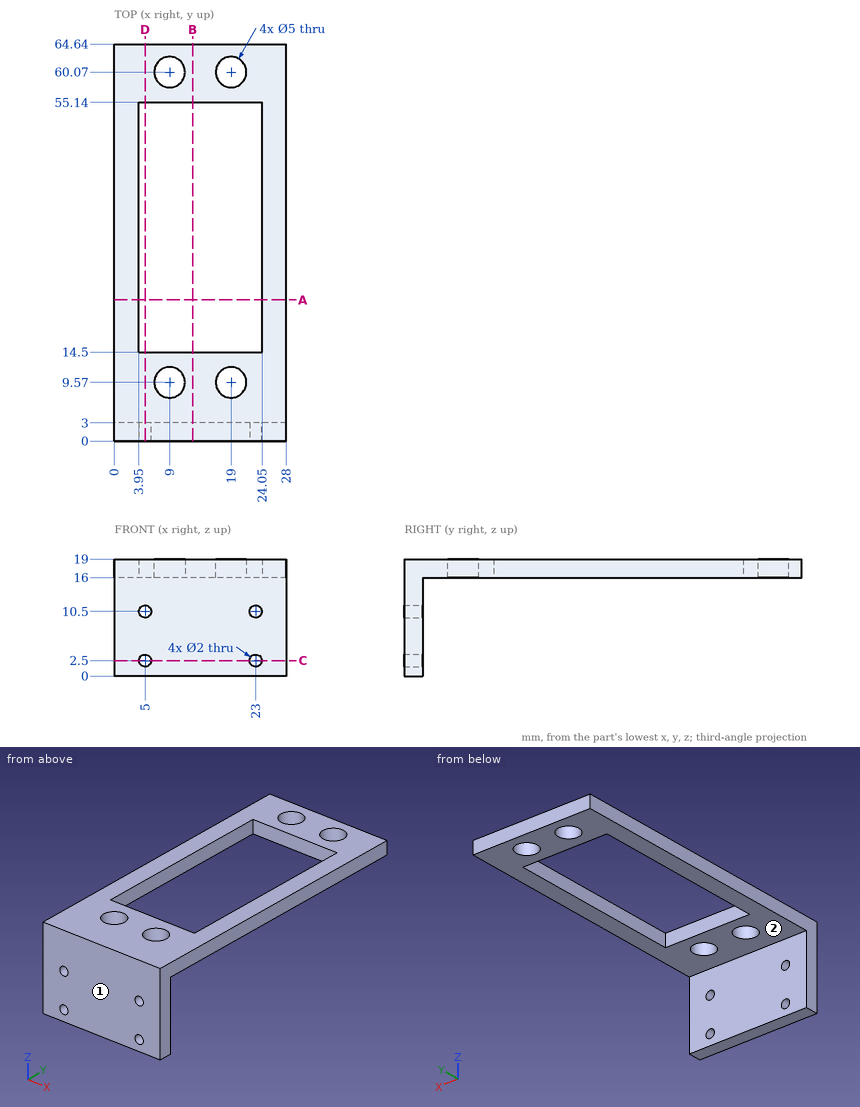
Answer from the drawing. Dimensions are ordinates in mm from the lowest x, y and z of the part. A direction names the side the tool comes from. Give positions to 0.01 mm unless a question says otherwise; leave off trailing zeros. Loops run counter-clockwise (first coordinate to the right, second up) from the corner with the lowest first, then second, coordinate; pieces in that order, holes last.
Item 1: For the marked faces 1 and 2, determine the directions among +Z, -Z, +X, -X, +Y, -Y from which every point of the face is accessible in a straight line to the end or side of a thin tool.
Item 2: Find the intervals of material crossed by line 1 along Z through (x, y) = (5, 0.7); line 2 along Y through (x, z) = (19, 17.45); line 3 along X through (y, z) = (10, 17), in increasing order.
Item 3: The part is cut by section A-A (y = 23). Write down the section's boundary in (x, z).
Item 4: The part is cut by section B-B (x = 12.75). Write down the section's boundary in (y, z), and give its area (3 significant figures).
Item 5: Each of these flat-tipped pins is pushed along its axis until it touches: pin 1 Ø4 at (x, y) = (19, 9.57) entering from -Z; pin 2 Ø6 at (x, y) = (9, 9.57) entering from -Z; pin 3 Ø5 at (x, z) = (12.5, 11.5) entering from +Y. Where does it stop, or does it pass through?
Item 6: The part is cut by section C-C (z = 2.5). Write down the section's boundary in (x, y), and give its area (3 significant figures).
Item 7: The part is cut by section D-D (x = 5). Write down the section's boundary in (y, z).
Taken from the geometry:
1. face 1: +Z, -Z, +X, -X, -Y
1. face 2: -Z, +X, -X, +Y
2. line 1: z = 0 to 1.5, 3.5 to 9.5, 11.5 to 19
2. line 2: y = 0 to 7.07, 12.07 to 14.5, 55.14 to 57.57, 62.57 to 64.64
2. line 3: x = 0 to 6.54, 11.46 to 16.54, 21.46 to 28
3. outline: (0, 16) - (3.95, 16) - (3.95, 19) - (0, 19) - close; (24.05, 16) - (28, 16) - (28, 19) - (24.05, 19) - close
4. outline: (0, 0) - (3, 0) - (3, 16) - (14.5, 16) - (14.5, 19) - (0, 19) - close; (55.14, 16) - (64.64, 16) - (64.64, 19) - (55.14, 19) - close
4. area: 120 mm2
5. pin 1: passes through
5. pin 2: stops at z = 16
5. pin 3: stops at y = 3
6. outline: (0, 0) - (4, 0) - (4, 3) - (0, 3) - close; (6, 0) - (22, 0) - (22, 3) - (6, 3) - close; (24, 0) - (28, 0) - (28, 3) - (24, 3) - close
6. area: 72.0 mm2
7. outline: (0, 0) - (3, 0) - (3, 1.5) - (0, 1.5) - close; (0, 3.5) - (3, 3.5) - (3, 9.5) - (0, 9.5) - close; (0, 11.5) - (3, 11.5) - (3, 16) - (14.5, 16) - (14.5, 19) - (0, 19) - close; (55.14, 16) - (64.64, 16) - (64.64, 19) - (55.14, 19) - close
